Design review of the part shown in the three views and the two pictorial views. Dimensions are in mm from the part's minimum x, y and z. Round coordinates to 2 decimals unless told otherwise and drop trailing zeros. Order: outer loops, then holes, each group sorted by start corner. A loop starts at its lowest first (then second) coordinate and runs counter-clockwise, first axis right, second up.
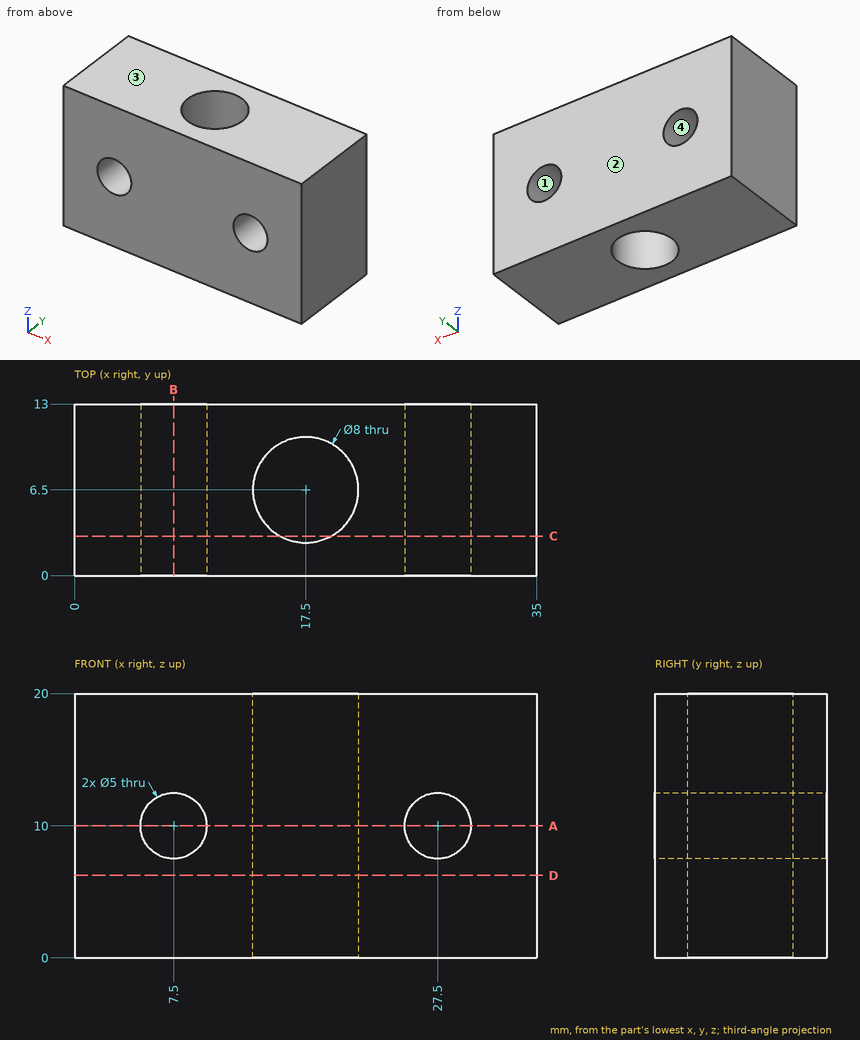
(1) Consider section C-C (y = 3). Write out the cut boundary in (x, z).
Data:
outline: (0, 0) - (15.56, 0) - (15.56, 20) - (0, 20) - close; (19.44, 0) - (35, 0) - (35, 20) - (19.44, 20) - close; hole circle Ø5 at (7.5, 10); hole circle Ø5 at (27.5, 10)
(2) Consider section D-D (z = 6.25). Write out the cut boundary in (x, y).
Data:
outline: (0, 0) - (35, 0) - (35, 13) - (0, 13) - close; hole circle Ø8 at (17.5, 6.5)
(3) Consider section B-B (x = 7.5). Write out the cut boundary in (y, z), and give its area (3 significant figures).
Data:
outline: (0, 0) - (13, 0) - (13, 7.5) - (0, 7.5) - close; (0, 12.5) - (13, 12.5) - (13, 20) - (0, 20) - close
area: 195 mm2
(4) To check wall thickness, follow probe 1 along Y at (x, z) = (17.5, 11.5); probe 2 along X at (y, z) = (8.75, 10); probe 3 along X at (y, z) = (7, 10.5). State the ranges of each line that lie inside material, in increasing order.
Data:
probe 1: y = 0 to 2.5, 10.5 to 13
probe 2: x = 0 to 5, 10 to 14.19, 20.81 to 25, 30 to 35
probe 3: x = 0 to 5.05, 9.95 to 13.53, 21.47 to 25.05, 29.95 to 35
(5) Draft analysis for pull direction Z (two halves, no side actions). For the marked faces 1, 2, 3 and 4, state which applies: pulls with the +Z half, pulls with the -Z half, needs draft (parallel to the pull), parting line crosses it, or undercut.
Data:
face 1: undercut
face 2: needs draft
face 3: pulls with the +Z half
face 4: undercut
(6) Consider section A-A (z = 10). Write out the cut boundary in (x, y).
Data:
outline: (0, 0) - (5, 0) - (5, 13) - (0, 13) - close; (10, 0) - (25, 0) - (25, 13) - (10, 13) - close; (30, 0) - (35, 0) - (35, 13) - (30, 13) - close; hole circle Ø8 at (17.5, 6.5)
